Answer from the drawing. Dimensions are ordinates in mm from the lowest x, y and z of the part. Round coordinates to 2 decimals unless told otherwise and drop trailing zeros. Loops run counter-clockwise (first coordinate to the right, second up) from the corner with the lowest first, then second, coordinate; pieces in that order, holes last.
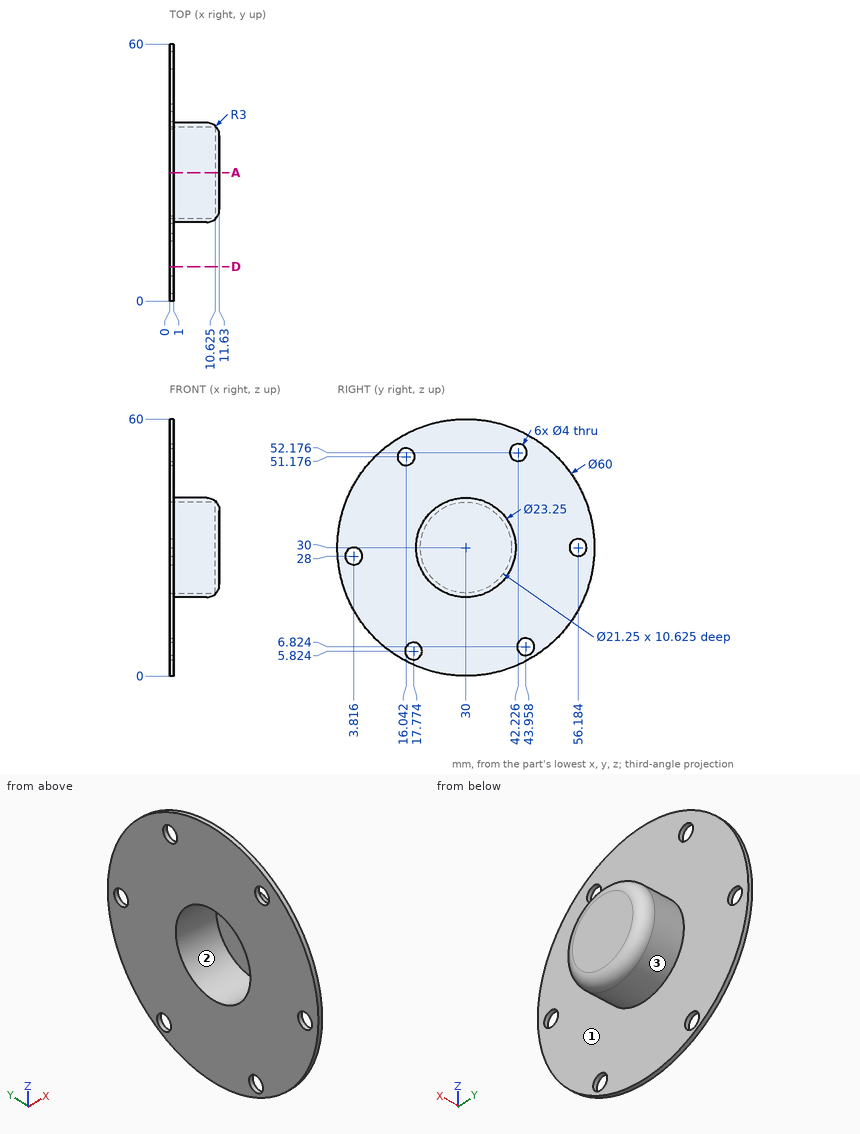
1. Given pin 1 (5 mm diameter, centred on y = 43.96, z = 6.82, fed in from -X); pin 2 (6 mm diameter, centred on y = 28, z = 32, fed in from -X) (3 decimals); pin 3 (1 mm diameter, centred on y = 49, z = 45, fed in from +X); pin 4 (1.5 mm diameter, centred on x = 6, y = 26.5, fed in from +Z) (1 decimal), each flat-ended and moving along its own axis, determine where each tip first touches the part or whether it passes through.
Answer key:
pin 1: stops at x = 0
pin 2: stops at x = 10.625
pin 3: stops at x = 1
pin 4: stops at z = 41.3
2. Find section D-D (y = 8). Write down the section's boundary in (x, z).
Answer key:
outline: (0, 9.6) - (1, 9.6) - (1, 50.4) - (0, 50.4) - close
3. Determine the mould class of the marked faces 1, 2 and 3 for opening direction Z: +Z half, -Z half, draft (parallel to the pull), parting line (faces both ways), or undercut.
Answer key:
face 1: draft
face 2: undercut
face 3: parting line
4. Find section A-A (y = 30). Write down the section's boundary in (x, z) (1 decimal).
Answer key:
outline: (0, 0) - (1, 0) - (1, 18.4) - (8.6, 18.4) arc R3 ccw to (11.6, 21.4) - (11.6, 38.6) arc R3 ccw to (8.6, 41.6) - (1, 41.6) - (1, 60) - (0, 60) - (0, 40.6) - (10.6, 40.6) - (10.6, 19.4) - (0, 19.4) - close
5. Consider probe 1 along X at (y, z) = (28, 14); probe 2 along X at (y, z) = (33.5, 36.5) (1 decimal); probe 3 along Y at (x, z) = (2, 35) (1 decimal). Determine where each line is inside the solid, lowest interval first.
Answer key:
probe 1: x = 0 to 1
probe 2: x = 10.6 to 11.6
probe 3: y = 19.5 to 20.6, 39.4 to 40.5
